Geometry: final body of the model. Coordinates: model frame, mm. A direction names the side the tool comes from. Give positions to 0.01 mm unless a question says otherwise; leave off trailing zeros. Write each loop counter-clockwise with the first axis right and the second up, starting at its lowest first coordinate (ties: lowest second). Pieces come first, ordered by that corner, then holes. Notation, with made-up numbers: (17, -4.75) - (28, -4.75) arc R21 cw to (28, 30.25) - close; hole circle Ø6 at (-4, 15). An arc over 180 degrees is marked (long way). Use CSV: the item, a comma, the result in double quotes. Start each with the question number.
(1) Draft query along X for faces 1 (the flat face through (200, -1, 13)), 2 (the flat face through (-3, 100, 13)), 3 (the cylindrical face through (90.26, 0.43, 84.56)), 4 (the cylindrical face through (-109.74, 0.43, 84.56)). Return one class per face: released by +X, released by -X, zero draft, split by the parting line, or undercut.
(2) Section C-C on y = 0. Output: boundary loops of the cut face in (x, z), and give its area (3 significant figures).
(3) Section D-D on x = 64. Output: boundary loops of the cut face in (y, z), and give its area (3 significant figures).
(4) Section B-B on z = 102. Output: boundary loops of the cut face in (x, y).
(5) First-contact query: pin 1 Ø4 at (x, y) = (66.5, 75.5) entering from +Z; pin 2 Ø8 at (y, z) = (13, 90) entering from +X; pin 3 Ø6 at (x, z) = (108.5, 36.5) entering from -Y. Flat tips, straight axial feed; report the tip coordinate or a pass-through.
(6) Reachability of faces 5 (the cylindrical face through (-1.269, 9.667, 84.56)), 6 (the flat face through (-3, 1, 0)) from +Z, -Z, +X, -X, +Y, -Y: full face, straight path, thin tool, end or side. Return the list, or none.
(7) Section A-A on x = 0. Output: boundary loops of the cut face in (y, z).
(8) Line query: probe 1 along Z at (x, y) = (156.5, -27.5); probe 2 along Y at (x, z) = (-102, 76); probe 3 along Y at (x, z) = (-95.5, 72.5). Output: solid intervals per line, ascending. Write a range as [from, to].
from build123d import *

# Parameters (mm, degrees)
F0_W     = 400
F0_H     = 200
F1_DEPTH = 25.4
F2_R     = 5.08
F3_R     = 9.75
F4_DEPTH = 120


with BuildPart() as f1:
    # F0 (on Top) → F1 (new body)
    with BuildSketch(Plane.XY):
        Rectangle(F0_W, F0_H)
    extrude(amount=F1_DEPTH)

    # F2
    f2_edges = [f1.edges().sort_by_distance(p)[0] for p in [
        (200, 100, 12.7),
        (200, -100, 12.7),
        (-200, 100, 12.7),
        (-200, -100, 12.7),
    ]]
    fillet(f2_edges, radius=F2_R)

    # F3 (on face) → F4 (join)
    with BuildSketch(Plane.XY.offset(25.4)):
        with Locations((-100, 0)):
            Circle(F3_R)
        Circle(F3_R)
        with Locations((100, 0)):
            Circle(F3_R)
    extrude(amount=F4_DEPTH)


solid = f1.part
Check values:
1,face 1,"released by +X"
1,face 2,"zero draft"
1,face 3,"undercut"
1,face 4,"undercut"
2,outline,"(-200, 0) - (200, 0) - (200, 25.4) - (109.75, 25.4) - (109.75, 145.4) - (90.25, 145.4) - (90.25, 25.4) - (9.75, 25.4) - (9.75, 145.4) - (-9.75, 145.4) - (-9.75, 25.4) - (-90.25, 25.4) - (-90.25, 145.4) - (-109.75, 145.4) - (-109.75, 25.4) - (-200, 25.4) - close"
2,area,"17,200 mm²"
3,outline,"(-100, 0) - (100, 0) - (100, 25.4) - (-100, 25.4) - close"
3,area,"5,080 mm²"
4,outline,"circle Ø19.5 at (-100, 0); circle Ø19.5 at (0, 0); circle Ø19.5 at (100, 0)"
5,pin 1,"stops at z = 25.4"
5,pin 2,"stops at x = 103.75"
5,pin 3,"stops at y = -8.05"
6,face 5,"+Z"
6,face 6,"-Z, +X, -X, +Y, -Y"
7,outline,"(-100, 0) - (100, 0) - (100, 25.4) - (9.75, 25.4) - (9.75, 145.4) - (-9.75, 145.4) - (-9.75, 25.4) - (-100, 25.4) - close"
8,probe 1,"z = [0, 25.4]"
8,probe 2,"y = [-9.54, 9.54]"
8,probe 3,"y = [-8.65, 8.65]"
